from build123d import *

# Parameters (mm, degrees)
SKETCH1_R           = 6
BOSS_EXTRUDE1_DEPTH = 30


with BuildPart() as part:
    # Sketch1 → Boss-Extrude1 (new body)
    with BuildSketch(Plane.XY):
        Circle(SKETCH1_R)
    boss_extrude1 = extrude(amount=-BOSS_EXTRUDE1_DEPTH)

    # Sketch5 → Tap Drill for M6x1.0 Tap1 (revolve, cut)
    with BuildSketch(Plane(origin=(0, 0, 0), x_dir=(0, -1, 0), z_dir=(1, 0, 0))):
        Polygon((0, 0), (0, 23.502151548), (2.5, 22), (2.5, 0), align=None)
    tap_drill_for_m6x1_0_tap1 = revolve(axis=Axis((0, 0, 6.35), (0, 0, -1)), mode=Mode.SUBTRACT)

    # Mirror1: Boss-Extrude1, Tap Drill for M6x1.0 Tap1 across plane
    add(boss_extrude1.mirror(Plane.XY.offset(-30)))
    add(tap_drill_for_m6x1_0_tap1.mirror(Plane.XY.offset(-30)), mode=Mode.SUBTRACT)


solid = part.part
The model under review builds one solid part; all positions refer to its coordinate system, in mm. A direction names the side the tool comes from. Round coordinates to 2 decimals unless told otherwise and drop trailing zeros. Write each loop counter-clockwise with the first axis right and the second up, starting at its lowest first coordinate (ties: lowest second). Pieces come first, ordered by that corner, then holes. Notation, with made-up numbers: (69.25, 52) -> (88.25, 52) arc R12 ccw to (88.25, 65) -> close; hole circle Ø9 at (87, 30). An arc over 180 degrees is marked (long way). Answer as a JSON object with one key per item and string values.
1. Machinability: for faces 1 (the face through (3, 0, -60)), 2 (the face through (2.44, 0.54, -10.85)), which of the approach directions +Z, -Z, +X, -X, +Y, -Y give a long, thin tool a straight path to every point of the face, cutting with its end or side? Answer none if there is none.
Results found:
{"face 1": "-Z, +X, -X, +Y, -Y", "face 2": "+Z"}
2. To check wall thickness, follow line 1 along Y through (x, z) = (0, -16.5); line 2 along Y through (x, z) = (-0.5, -47.5). State the ranges of each line that lie inside material, in increasing order.
Results found:
{"line 1": "y = -6 to -2.5, 2.5 to 6", "line 2": "y = -5.98 to -2.45, 2.45 to 5.98"}
3. We need section A-A on z = -48. State the section outline as (x, y) points, and give its area (3 significant figures).
Results found:
{"outline": "circle Ø12 at (0, 0); hole circle Ø5 at (0, 0)", "area": "93.5 mm^2"}
4. The part is to be moulded in two halves that separate along X. For faces 3 (the face through (2.44, 0.54, -49.15)), 4 (the face through (-6, 0, -30)), 5 (the face through (3, 0, 0)), 6 (the face through (0.424, 0.094, -23.241)), say which applies: pulls with the +X half, pulls with the -X half, needs draft (parallel to the pull), parting line crosses it, or undercut.
Results found:
{"face 3": "undercut", "face 4": "parting line crosses it", "face 5": "needs draft", "face 6": "undercut"}
5. We need section C-C on y = -5. State the section outline as (x, z) points, and give its area (3 significant figures).
Results found:
{"outline": "(-3.32, -60) -> (3.32, -60) -> (3.32, 0) -> (-3.32, 0) -> close", "area": "398 mm^2"}
6. We need section B-B on z = -27. State the section outline as (x, y) points.
Results found:
{"outline": "circle Ø12 at (0, 0)"}
7. We need section D-D on z = -37. State the section outline as (x, y) points.
Results found:
{"outline": "circle Ø12 at (0, 0); hole circle Ø1.67 at (0, 0)"}
8. Clearance check with flat-ended pins moving along their axes: pin 1 (6 mm diameter, centred on y = 4, z = -28.5, fed in from +X); pin 2 (1 mm diameter, centred on y = 2.5, z = -26.5, fed in from +X); pin 3 (3 mm diameter, centred on x = -4.5, z = -41.5, fed in from -Y). State where each tip first meets the part, or that it passes through.
Results found:
{"pin 1": "stops at x = 5.92", "pin 2": "stops at x = 5.66", "pin 3": "stops at y = -5.2"}
